Geometry: see drawing. Coordinates: mm, zero at the bounding-box minimum. Give positions to 0.01 mm unless a question says otherwise; leave off trailing zeros. Write each loop counter-clockwise with the first axis right and the second up, starting at its lowest first coordinate (ties: lowest second). Pieces come first, ordered by that corner, then holes. Notation, with made-up numbers: M -4,88.25 L 13,88.25 A18 ccw 13,108.25 Z; hole C 40,5.25 d4. An arc over 180 degrees is marked long. Use one line per item in the form item = value. Start each with the question number.
Item 1: Section query C-C on y = 0.6. Return loops of the section in (x, z), then the cut area to 3 significant figures.
Item 2: Section query B-B on z = 12.25. Return loops of the section in (x, y).
Item 3: Material intervals for line 1 along Z through (x, y) = (12.25, 1.1); line 2 along X through (y, z) = (1.4, 12.25); line 3 along Z through (x, y) = (10.25, 1.9), sorted ascending. Write a range as from..to.
Item 4: Contact query for flat-ended pins moving along their axis: P1, Ø1.8, axis at x = 12.25, z = 17.21, coming from the -Y side; P2, Ø10, axis at x = 12.25, z = 12.25, coming from the -Y side. Output: stop coordinate, or through.
Item 5: Section query A-A on x = 12.25. Return loops of the section in (y, z), then the cut area to 3 significant figures.
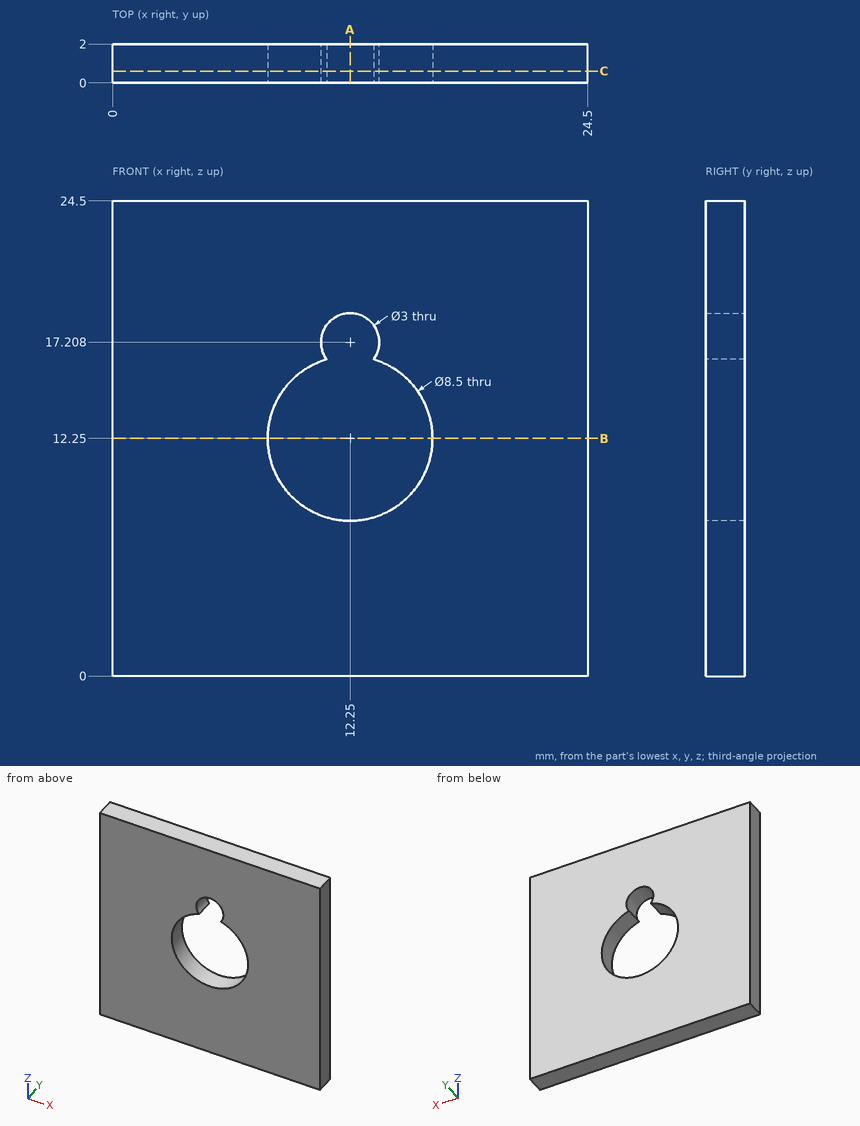
Answer sheet:
q1.outline = M 0,0 L 24.5,0 L 24.5,24.5 L 0,24.5 Z; hole M 11.04,16.32 A4.25 ccw long 13.46,16.32 A1.5 ccw long Z
q1.area = 538 mm2
q2.outline = M 0,0 L 8,0 L 8,2 L 0,2 Z; M 16.5,0 L 24.5,0 L 24.5,2 L 16.5,2 Z
q3.line_1 = 0..8, 18.71..24.5
q3.line_2 = 0..8, 16.5..24.5
q3.line_3 = 0..8.5, 16..24.5
q4.P1 = through
q4.P2 = 0
q5.outline = M 0,0 L 2,0 L 2,8 L 0,8 Z; M 0,18.71 L 2,18.71 L 2,24.5 L 0,24.5 Z
q5.area = 27.6 mm2
